Verification items for the finished model (mm, model axes). Coordinates: 2 decimals unless noted, no trailing zeros. Loops run counter-clockwise (first coordinate to the right, second up) from the corner with the lowest first, then second, coordinate; pieces in that order, holes last. Notation, with made-up numbers: (66, -2) -> (96, -2) arc R12 cw to (96, 9) -> close; hole circle Ø11 at (-22.5, -19). An arc over 180 degrees is marked (long way). Answer as a JSON object with one key per item and string values. Group by question number.
Q1. Release check for a two-part mould opening along X. For faces 1 (the conical face through (-9.1, 0.1, 1.6)), 2 (the flat face through (6, 0, -2)), 3 (the cylindrical face through (-1.08, -4.88, -0.02)) record: released by +X, released by -X, zero draft, split by the parting line, or undercut.
Q2. Gauge pin test, flat end, axial feed: pin 1 Ø2 at (y, z) = (1, -1) entering from +X. Record the tip position at first contact, or that the pin passes through.
Q3. Cross-section at A-A on x = 0. Record the boundary of the cut face in (y, z).
Q4. Scan lines: L1, parallel to Y at x = 0, z = 0.2; L2, parallel to Y at x = -2.5, z = 0.65; L3, parallel to X at y = 4.25, z = 1.6. Record each from-to range of solid material in increasing order.
```python
from build123d import *

# Parameters (mm, degrees)
BOSS_EXTRUDE1_DEPTH = 2
SKETCH2_R           = 5
CUT_EXTRUDE1_DEPTH  = 14.820274961
CHAMFER1_SIZE       = 0.5


with BuildPart() as part:
    # Sketch1 → Boss-Extrude1 (new, symmetric)
    with BuildSketch(Plane.XY):
        Polygon((-10, 0), (-5, -8.660254038), (5, -8.660254038), (10, 0), (5, 8.660254038), (-5, 8.660254038), align=None)
    extrude(amount=BOSS_EXTRUDE1_DEPTH, both=True)

    # Sketch2 → Cut-Extrude1 (cut, through all)
    with BuildSketch(Plane.XY.offset(-2)):
        Circle(SKETCH2_R)
    extrude(amount=CUT_EXTRUDE1_DEPTH, mode=Mode.SUBTRACT)

    # Sketch8 → Cut-Revolve1 (revolve, cut)
    with BuildSketch(Plane(origin=(0, 0, 0), x_dir=(1, 0, 0), z_dir=(0, 1, 0))):
        Polygon((-8.6, -2.1), (-10.1, -2.1), (-10.1, -0.6), align=None)
    cut_revolve1 = revolve(axis=Axis((0, 0, -7.705), (0, 0, 1)), mode=Mode.SUBTRACT)

    # Mirror1: Cut-Revolve1 across plane
    add(cut_revolve1.mirror(Plane.XY), mode=Mode.SUBTRACT)

    # Chamfer1
    chamfer1_edges = [part.edges().sort_by_distance(p)[0] for p in [
        (-5, 0, -2),
        (-5, 0, 2),
    ]]
    chamfer(chamfer1_edges, length=CHAMFER1_SIZE)


solid = part.part
```
Computed values:
{
 "1": {"face 1": "released by -X", "face 2": "zero draft", "face 3": "undercut"},
 "2": {"pin 1": "stops at x = 9.98"},
 "3": {"outline": "(-8.66, -2) -> (-5.5, -2) -> (-5, -1.5) -> (-5, 1.5) -> (-5.5, 2) -> (-8.66, 2) -> close; (5, -1.5) -> (5.5, -2) -> (8.66, -2) -> (8.66, 2) -> (5.5, 2) -> (5, 1.5) -> close"},
 "4": {"L1": "y = -8.66 to -5, 5 to 8.66", "L2": "y = -8.66 to -4.33, 4.33 to 8.66", "L3": "x = -7.55 to -2.82, 2.82 to 7.55"}
}
